Work out the finished part from the listing and answer in its coordinate system (mm). A direction names the side the tool comes from. Give positions to 0.01 mm unless a question says otherwise; leave off trailing zeros. Order: outer loops, then holes, each group sorted by start corner. A loop starts at its lowest first (then second) coordinate and runs counter-clockwise, first axis right, second up. Notation, with made-up numbers: (72, -18.75) - (120, -18.75) arc R22 ccw to (120, 5.25) - close; hole circle Ø10 at (-16, 70). An arc over 180 degrees is marked (long way). Put each result on its own line as item: value.
```python
from build123d import *

# Parameters (mm, degrees)
SKETCH_1_W                       = 60
SKETCH_1_H                       = 60
SKETCH_1_R                       = 1.65
SKETCH_1_R_2                     = 19.5
SKETCH_1_R_3                     = 2
SM_BASE_FLANGE_1_DEPTH           = 4
SKETCH_4_W                       = 40
SKETCH_4_H                       = 4
EXTRUDE_1_DEPTH                  = 0.1
SM_EDGE_FLANGE_1_DEPTH           = 40
SM_EDGE_FLANGE_2_STRIP_W         = 18.4
SM_EDGE_FLANGE_2_STRIP_H         = 4
SM_EDGE_FLANGE_2_STRIP_CUT_DEPTH = 40
SM_EDGE_FLANGE_2_DEPTH           = 40
FILLET_1_R                       = 2
SKETCH_11_R                      = 12.5
CUT_EXTRUDE_1_DEPTH              = 10
FILLET_2_R                       = 20


# Sheet-metal steps are written as plain solids
with BuildPart() as part:
    # Sketch 1 → Базовая кромка1 (new body)
    with BuildSketch(Plane(origin=(0, 0, 0), x_dir=(1, 0, 0), z_dir=(0, 1, 0))):
        with Locations((-9.094903125, 3.781032797)):
            Rectangle(SKETCH_1_W, SKETCH_1_H)
        with Locations(Location((-32.594903125, 27.281032797, 0), (0, 0, 270))):
            Circle(SKETCH_1_R, mode=Mode.SUBTRACT)
        with Locations(Location((14.405096875, 27.281032797, 0), (0, 0, 270))):
            Circle(SKETCH_1_R, mode=Mode.SUBTRACT)
        with Locations(Location((-32.594903125, -19.718967203, 0), (0, 0, 270))):
            Circle(SKETCH_1_R, mode=Mode.SUBTRACT)
        with Locations(Location((14.405096875, -19.718967203, 0), (0, 0, 270))):
            Circle(SKETCH_1_R, mode=Mode.SUBTRACT)
        with Locations(Location((-9.094903125, 3.781032797, 0), (0, 0, 270))):
            Circle(SKETCH_1_R_2, mode=Mode.SUBTRACT)
        with Locations(Location((-34.094903125, 3.781032797, 0), (0, 0, 270))):
            Circle(SKETCH_1_R_3, mode=Mode.SUBTRACT)
        with Locations(Location((15.905096875, 3.781032797, 0), (0, 0, 270))):
            Circle(SKETCH_1_R_3, mode=Mode.SUBTRACT)
        with Locations(Location((-9.094903125, 28.781032797, 0), (0, 0, 270))):
            Circle(SKETCH_1_R_3, mode=Mode.SUBTRACT)
        with Locations(Location((-9.094903125, -21.218967203, 0), (0, 0, 270))):
            Circle(SKETCH_1_R_3, mode=Mode.SUBTRACT)
    extrude(amount=-SM_BASE_FLANGE_1_DEPTH)

    # Эскиз4 → Бобышка-Вытянуть1 (add)
    with BuildSketch(Plane.ZY.offset(39.094903125)):
        with Locations((-3.781032797, -2)):
            Rectangle(SKETCH_4_W, SKETCH_4_H)
    extrude(amount=EXTRUDE_1_DEPTH)

    # Ребро-кромка1 section (across the edge) → Ребро-кромка1 (add)
    with BuildSketch(Plane(origin=(-40.394903125, 0, -23.781032797), x_dir=(1, 0, 0), z_dir=(0, 0, 1))):
        with BuildLine():
            Line((-4, 1.2), (-4, 30))
            Line((-4, 30), (0, 30))
            Line((0, 30), (0, 1.2))
            ThreePointArc((0, 1.2), (0.351471863, 0.351471863), (1.2, 0))
            Line((1.2, 0), (1.2, -4))
            ThreePointArc((1.2, -4), (-2.476955262, -2.476955262), (-4, 1.2))
        make_face()
    extrude(amount=SM_EDGE_FLANGE_1_DEPTH)

    # Ребро-кромка2 strip (across the edge) → Ребро-кромка2 strip cut (cut)
    with BuildSketch(Plane(origin=(-44.394903125, 30, 16.218967203), x_dir=(0, -1, 0), z_dir=(0, 0, -1))):
        with Locations((-8, -2)):
            Rectangle(SM_EDGE_FLANGE_2_STRIP_W, SM_EDGE_FLANGE_2_STRIP_H)
    extrude(amount=SM_EDGE_FLANGE_2_STRIP_CUT_DEPTH, mode=Mode.SUBTRACT)

    # Ребро-кромка2 section (across the edge) → Ребро-кромка2 (add)
    with BuildSketch(Plane(origin=(-44.394903125, 30, 16.218967203), x_dir=(0, -1, 0), z_dir=(0, 0, -1))):
        with BuildLine():
            Line((-4, 1.2), (-4, 40))
            Line((-4, 40), (0, 40))
            Line((0, 40), (0, 1.2))
            ThreePointArc((0, 1.2), (0.351471863, 0.351471863), (1.2, 0))
            Line((1.2, 0), (1.2, -4))
            ThreePointArc((1.2, -4), (-2.476955262, -2.476955262), (-4, 1.2))
        make_face()
    extrude(amount=SM_EDGE_FLANGE_2_DEPTH)

    # Скругление1
    fillet_1_edges = [part.edges().sort_by_distance(p)[0] for p in [
        (-39.094903125, -2, -33.781032797),
        (20.905096875, -2, -33.781032797),
        (20.905096875, -2, 26.218967203),
        (-39.094903125, -2, 26.218967203),
    ]]
    fillet(fillet_1_edges, radius=FILLET_1_R)

    # Эскиз11 → Вырез-Вытянуть1 (cut)
    with BuildSketch(Plane(origin=(0, 34, 0), x_dir=(1, 0, 0), z_dir=(0, 1, 0))):
        with Locations(Location((-64.394903125, 3.781032797, 0), (0, 0, 270))):
            Circle(SKETCH_11_R)
    extrude(amount=-CUT_EXTRUDE_1_DEPTH, mode=Mode.SUBTRACT)

    # Скругление2
    fillet_2_edges = [part.edges().sort_by_distance(p)[0] for p in [
        (-84.394903125, 32, -23.781032797),
        (-84.394903125, 32, 16.218967203),
    ]]
    fillet(fillet_2_edges, radius=FILLET_2_R - 0.0001)  # a hair under: the kernel refuses the full size


solid = part.part
```
(1) A tool of negligible diameter and unlimited length cuts with its end or side. For faces 1 (the face through (-39.095, -2, 20)), 2 (the face through (-40.395, 15, -4)), 3 (the face through (20.905, -2, -3)), from which of +Z, -Z, +X, -X, +Y, -Y can it reach the whole face along a straight path? Write none if from no direction.
Geometry check:
face 1: +Z, -X, +Y, -Y
face 2: +Z, -Z, +X, +Y
face 3: +Z, -Z, +X, +Y, -Y
(2) Section B-B, the plane x = 0 is taken. Write down the section's boundary in (y, z), then the cut area to 3 significant figures.
Geometry check:
outline: (-4, -33.78) - (0, -33.78) - (0, -21.03) - (-4, -21.03) - close; (-4, 13.47) - (0, 13.47) - (0, 26.22) - (-4, 26.22) - close
area: 102 mm²
(3) Section A-A, the plane z = -7.5 is taken. Write down the section's boundary in (x, y).
Geometry check:
outline: (-84.05, 30) - (-76.33, 30) - (-76.33, 34) - (-84.05, 34) - close; (-52.46, 30) - (-45.59, 30) arc R1.2 cw to (-44.39, 28.8) - (-44.39, 1.2) arc R5.2 ccw to (-39.19, -4) - (-28.24, -4) - (-28.24, 0) - (-39.19, 0) arc R1.2 cw to (-40.39, 1.2) - (-40.39, 28.8) arc R5.2 ccw to (-45.59, 34) - (-52.46, 34) - close; (10.05, -4) - (20.91, -4) - (20.91, 0) - (10.05, 0) - close
(4) Section D-D, the plane x = -15 is taken. Write down the section's boundary in (y, z), then the cut area to 3 significant figures.
Geometry check:
outline: (-4, -33.78) - (0, -33.78) - (0, -22.37) - (-4, -22.37) - close; (-4, 14.8) - (0, 14.8) - (0, 26.22) - (-4, 26.22) - close
area: 91.3 mm²
(5) Straight lines are drawn through the part: line 1 (Z direction, x = 13, y = -2); line 2 (Y direction, x = -37, z = 12); line 3 (X direction, y = 24, z = -11). For each, find the intervals that lie inside material, in ascending order.
Geometry check:
line 1: z = -33.78 to -28.15, -26.42 to 18.85, 20.58 to 26.22
line 2: y = -4 to 0
line 3: x = -44.39 to -40.39
(6) Determine the mould class of faces 4 (the face through (-39.095, -2, -28)), 5 (the face through (20.3, -2.03, 25.65)), 6 (the face through (-9.01, -1.97, -30.78)) for opening direction X: pulls with the +X half, pulls with the -X half, needs draft (parallel to the pull), parting line crosses it, or undercut.
Geometry check:
face 4: pulls with the -X half
face 5: pulls with the +X half
face 6: undercut
(7) Given pin 1 (1.5 mm diameter, centred on y = 17, z = -8.5, fed in from -X); pin 2 (5 mm diameter, centred on x = -37, z = -11, fed in from +Y); pin 3 (14 mm diameter, centred on y = 14, z = -5.5, fed in from +X), each flat-ended and moving along its own axis, determine where each tip first touches the part or whether it passes through.
Geometry check:
pin 1: stops at x = -44.39
pin 2: stops at y = 0.04
pin 3: stops at x = -40.39
(8) Section C-C, the plane z = 10.5 is taken. Write down the section's boundary in (x, y), then the cut area to 3 significant figures.
Geometry check:
outline: (-78.4, 30) - (-45.59, 30) arc R1.2 cw to (-44.39, 28.8) - (-44.39, 1.2) arc R5.2 ccw to (-39.19, -4) - (-22.37, -4) - (-22.37, 0) - (-39.19, 0) arc R1.2 cw to (-40.39, 1.2) - (-40.39, 28.8) arc R5.2 ccw to (-45.59, 34) - (-78.4, 34) - close; (4.18, -4) - (20.91, -4) - (20.91, 0) - (4.18, 0) - close
area: 416 mm²
